from build123d import *

# Parameters (mm, degrees)
SKETCH1_R           = 30
SKETCH1_R_2         = 20
BOSS_EXTRUDE1_DEPTH = 2
SKETCH2_R           = 20
SKETCH2_R_2         = 18
BOSS_EXTRUDE2_DEPTH = 7
SKETCH3_R           = 18
SKETCH3_R_2         = 16
BOSS_EXTRUDE3_DEPTH = 25


with BuildPart() as part:
    # Sketch1 → Boss-Extrude1 (new body)
    with BuildSketch(Plane(origin=(0, 0, 0), x_dir=(1, 0, 0), z_dir=(0, 1, 0))):
        Circle(SKETCH1_R)
        Circle(SKETCH1_R_2, mode=Mode.SUBTRACT)
    extrude(amount=BOSS_EXTRUDE1_DEPTH)

    # Sketch2 → Boss-Extrude2 (add)
    with BuildSketch(Plane(origin=(0, 0, 0), x_dir=(1, 0, 0), z_dir=(0, 1, 0))):
        Circle(SKETCH2_R)
        Circle(SKETCH2_R_2, mode=Mode.SUBTRACT)
    extrude(amount=BOSS_EXTRUDE2_DEPTH)

    # Sketch3 → Boss-Extrude3 (add)
    with BuildSketch(Plane(origin=(0, 0, 0), x_dir=(1, 0, 0), z_dir=(0, 1, 0))):
        Circle(SKETCH3_R)
        Circle(SKETCH3_R_2, mode=Mode.SUBTRACT)
    extrude(amount=BOSS_EXTRUDE3_DEPTH)


solid = part.part
Input: part model. Units: mm. Frame: model coordinates. A direction names the side the tool comes from. Coordinates: 2 decimals unless noted, no trailing zeros. Loops run counter-clockwise (first coordinate to the right, second up) from the corner with the lowest first, then second, coordinate; pieces in that order, holes last. Notation, with made-up numbers: (29.25, 77) - (67.25, 77) arc R20 ccw to (67.25, 103) - close; hole circle Ø9 at (80, -20.5). An arc over 180 degrees is marked (long way). Answer in a Markdown table with one row per item. Add a question column.
Item 1: Section query D-D on x = -21. Return the cut outline in (y, z), then the cut area to 3 significant figures.
Item 2: Section query A-A on x = 0. Return the cut outline in (y, z), then the cut area to 3 significant figures.
Item 3: Section query C-C on y = 6. Return the cut outline in (x, z).
Item 4: Section query B-B on z = -3. Return the cut outline in (x, y), then the cut area to 3 significant figures.
Item 5: Line query: line 1 along Z through (x, y) = (0, 18.25); line 2 along X through (y, z) = (6, 0). Output: solid intervals per line, ascending. Write a range as [from, to].
Item 6: Access query for faces 4 (the flat face through (6, 2, 20)), 5 (the cylindrical face through (-29.97, 0.99, -1.32)). Directions: +Z, -Z, +X, -X, +Y, -Y. A direction counts if a zero-diameter tool reaches every point of the face in a straight line with its end or side. Return the directions, or none.
Item 7: Contact query for flat-ended pins moving along their axis: P1, Ø2, axis at x = 17, z = -20, coming from the +Y side; P2, Ø4, axis at y = 19.5, z = 16.5, coming from the -X side; P3, Ø12, axis at x = 3, y = 17.5, coming from the +Z side. Output: stop coordinate, or through.
Item 8: Mould query, pull axis X, two halves, no side actions, for faces 1 (the flat face through (13, 0, 13)), 2 (the cylindrical face through (-4.336, 4.465, 19.524)), 3 (the cylindrical face through (-3.47, 12.32, 15.62)). Classes: released by +X, released by -X, zero draft, split by the parting line, or undercut.
Recorded:
| question | item | result |
|---|---|---|
| 1 | outline | (0, -21.42) - (2, -21.42) - (2, 21.42) - (0, 21.42) - close |
| 1 | area | 85.7 mm^2 |
| 2 | outline | (0, -30) - (2, -30) - (2, -20) - (7, -20) - (7, -18) - (25, -18) - (25, -16) - (0, -16) - close; (0, 16) - (25, 16) - (25, 18) - (7, 18) - (7, 20) - (2, 20) - (2, 30) - (0, 30) - close |
| 2 | area | 168 mm^2 |
| 3 | outline | circle Ø40 at (0, 0); hole circle Ø32 at (0, 0) |
| 4 | outline | (-29.85, 0) - (-15.72, 0) - (-15.72, 25) - (-17.75, 25) - (-17.75, 7) - (-19.77, 7) - (-19.77, 2) - (-29.85, 2) - close; (15.72, 0) - (29.85, 0) - (29.85, 2) - (19.77, 2) - (19.77, 7) - (17.75, 7) - (17.75, 25) - (15.72, 25) - close |
| 4 | area | 170 mm^2 |
| 5 | line 1 | [-18, -16], [16, 18] |
| 5 | line 2 | [-20, -16], [16, 20] |
| 6 | face 4 | +Y |
| 6 | face 5 | +Y, -Y |
| 7 | P1 | y = 2 |
| 7 | P2 | x = -10.67 |
| 7 | P3 | z = 18 |
| 8 | face 1 | zero draft |
| 8 | face 2 | split by the parting line |
| 8 | face 3 | undercut |
